from build123d import *

# Parameters (mm, degrees)
SKETCH2_R          = 1.7272
CUT_EXTRUDE1_DEPTH = 39.1
SKETCH3_R          = 35.433
SKETCH3_R_2        = 31.242
CUT_EXTRUDE2_DEPTH = 3.175
SKETCH4_R          = 1.03251
CUT_EXTRUDE3_DEPTH = 3.175
CIRPATTERN1_COUNT  = 9
SKETCH5_R          = 3.175
CUT_EXTRUDE4_DEPTH = 9.525
FILLET1_R          = 1.27


with BuildPart() as part:
    # Sketch1 → Revolve1 (revolve)
    with BuildSketch(Plane.XY):
        with BuildLine():
            Line((3.94335, 7.43458), (38.1, 7.43458))
            Line((38.1, 7.43458), (38.1, -8.82142))
            Line((38.1, -8.82142), (22.6695, -8.82142))
            Line((22.6695, -8.82142), (22.6695, -7.8105))
            Line((22.6695, -7.8105), (21.1455, -7.8105))
            Line((21.1455, -7.8105), (21.1455, -8.8265))
            Line((21.1455, -8.8265), (10.9855, -8.8265))
            Line((10.9855, -8.8265), (10.9855, -6.391948453))
            ThreePointArc((10.9855, -6.391948453), (10.570616467, -5.000733157), (9.4615, -4.064))
            Line((9.4615, -4.064), (3.94335, 0))
            Line((3.94335, 0), (3.94335, 7.43458))
        make_face()
    revolve(axis=Axis((0, 101.60464546, 0), (0, 1, 0)))

    # Sketch2 → Cut-Extrude1 (cut, through all)
    with BuildSketch(Plane(origin=(0, 0, 0), x_dir=(0, 0, -1), z_dir=(1, 0, 0))):
        with Locations((0, -2.21742)):
            Circle(SKETCH2_R)
    extrude(amount=CUT_EXTRUDE1_DEPTH, mode=Mode.SUBTRACT)

    # Sketch3 → Cut-Extrude2 (cut)
    with BuildSketch(Plane(origin=(0, 7.43458, 0), x_dir=(1, 0, 0), z_dir=(0, 1, 0))):
        Circle(SKETCH3_R)
        Circle(SKETCH3_R_2, mode=Mode.SUBTRACT)
    extrude(amount=-CUT_EXTRUDE2_DEPTH, mode=Mode.SUBTRACT)

    # Sketch4 → Cut-Extrude3 (cut)
    with BuildSketch(Plane(origin=(0, -8.82142, 0), x_dir=(-1, 0, 0), z_dir=(0, -1, 0))):
        with Locations((-13.97, 24.196749782)):
            Circle(SKETCH4_R)
    cut_extrude3 = extrude(amount=-CUT_EXTRUDE3_DEPTH, mode=Mode.SUBTRACT)

    # CirPattern1: Cut-Extrude3 ×9 about axis
    cirpattern1_axis = Axis((0, 0, 0), (0, 1, 0))
    for i in range(1, CIRPATTERN1_COUNT):
        add(cut_extrude3.rotate(cirpattern1_axis, i * 360 / CIRPATTERN1_COUNT), mode=Mode.SUBTRACT)

    # Sketch5 → Cut-Extrude4 (cut)
    with BuildSketch(Plane(origin=(38.1, 0, 0), x_dir=(0, 0, -1), z_dir=(1, 0, 0))):
        with Locations((0, -2.21742)):
            Circle(SKETCH5_R)
    extrude(amount=-CUT_EXTRUDE4_DEPTH, mode=Mode.SUBTRACT)

    # Fillet1
    fillet1_edges = [part.edges().sort_by_distance(p)[0] for p in [
        (-3.94335, 0, 0),
    ]]
    fillet(fillet1_edges, radius=FILLET1_R)


solid = part.part
Read the model definition and answer for the solid it produces. Units are mm, in the model's axes. A direction names the side the tool comes from. Give positions to 0.01 mm unless a question says otherwise; leave off trailing zeros. Write each loop counter-clockwise with the first axis right and the second up, starting at its lowest first coordinate (ties: lowest second). Pieces come first, ordered by that corner, then holes. Notation, with made-up numbers: (-22, 53.25) - (2, 53.25) arc R19 cw to (2, 75.25) - close; hole circle Ø4 at (17.25, 85.25). An arc over 180 degrees is marked (long way). Answer in a Markdown table with one row per item. Add a question column.
Item 1: Flat-ended cylindrical pins translate along their axes: P1, Ø1.7, axis at x = -22, z = -18, coming from the -Y side; P2, Ø8, axis at x = -26, y = -3.5, coming from the +Z side; P3, Ø0.6, axis at x = 26.5, z = -10, coming from the -Y side; P4, Ø4.5, axis at x = 0, z = 0, coming from the -Y side. Find the tip coordinate at first contact, or state that the pin passes through.
Item 2: A tool of negligible diameter and unlimited length cuts with its end or side. For faces 4 (the face through (9, -8.826, 9)), 5 (the face through (-4.72, -7.26, 26.49)), 6 (the face through (-4.067, 5.869, -30.976)), 7 (the face through (16.4, -0.5, 0.2)), from which of +Z, -Z, +X, -X, +Y, -Y can it reach the whole face along a straight path? Write none if from no direction.
Item 3: Section C-C, the plane x = -24 is taken. Write down the section's boundary in (y, z).
Item 4: Section A-A, the plane x = 33 is taken. Write down the section's boundary in (y, z) (3 decimals).
Item 5: Section D-D, the plane z = 0 is taken. Count the separate pieces of the cut face and the enclosed holes in it, and give its area (3 significant figures).
Item 6: Determine the mould class of faces 1 (the face through (33.404, -5.317, 0.688)), 2 (the face through (12.985, -7.256, 23.887)), 3 (the face through (-21, -5.646, 18)) for opening direction Y: pulls with the +Y half, pulls with the -Y half, needs draft (parallel to the pull), parting line crosses it, or undercut.
Item 7: Find the intervals of material crossed by L1, parallel to X at y = 5.2, z = 0; L2, parallel to Z at x = 13.97, y = -7.1; L3, parallel to Z at x = 0, y = -8.45, in increasing order.
Item 8: Section B-B, the plane y = 3 is taken. Write down the section's boundary in (x, z).
Recorded:
| question | item | result |
|---|---|---|
| 1 | P1 | stops at y = -8.82 |
| 1 | P2 | stops at z = 31.11 |
| 1 | P3 | stops at y = -5.65 |
| 1 | P4 | passes through |
| 2 | face 4 | +Z, -Z, +X, -X, -Y |
| 2 | face 5 | -Y |
| 2 | face 6 | +Y |
| 2 | face 7 | +X |
| 3 | outline | (-8.82, -29.59) - (7.43, -29.59) - (7.43, -26.07) - (4.26, -26.07) - (4.26, -20) - (7.43, -20) - (7.43, 20) - (4.26, 20) - (4.26, 26.07) - (7.43, 26.07) - (7.43, 29.59) - (-8.82, 29.59) - close |
| 4 | outline | (-8.821, -19.042) - (7.435, -19.042) - (7.435, -12.903) - (4.26, -12.903) - (4.26, 12.903) - (7.435, 12.903) - (7.435, 19.042) - (-8.821, 19.042) - close; hole circle Ø6.35 at (-2.217, 0) |
| 5 | separate pieces | 3 |
| 5 | enclosed holes | 0 |
| 5 | area | 852 mm2 |
| 6 | face 1 | undercut |
| 6 | face 2 | needs draft |
| 6 | face 3 | pulls with the -Y half |
| 7 | L1 | x = -38.1 to -35.43, -31.24 to -3.94, 3.94 to 31.24, 35.43 to 38.1 |
| 7 | L2 | z = -35.45 to -25.23, -23.16 to 23.16, 25.23 to 35.45 |
| 7 | L3 | z = -38.1 to -22.67, -21.15 to -10.99, 10.99 to 21.15, 22.67 to 38.1 |
| 8 | outline | circle Ø76.2 at (0, 0); hole circle Ø7.89 at (0, 0) |
